For this review, use the dimensioned drawing (mm, ordinates from the lowest corner) and the shaded views. Round coordinates to 2 decimals unless told otherwise and drop trailing zeros. Write each loop counter-clockwise with the first axis right and the second up, starting at its lowest first coordinate (ties: lowest second). Pieces come first, ordered by that corner, then holes. Notation, with made-up numbers: M 27.5,34 L 79.5,34 A19 ccw 79.5,41 Z; hole C 21.5,78 d5. An arc over 180 degrees is marked long. One line per question, with ' | ' between items. Start each with the question number.
Item 1: For L1, parallel to Y at x = 2.25, z = 0.75 (1 decimal); L2, parallel to Z at x = 1, y = 1.5; L3, parallel to Z at x = 0.5, y = 2.25 (1 decimal), list the stretches that pass through material, from the lowest coordinate up.
Item 2: Insertion check: pin 1 Ø2.5 at (x, y) = (3.175, 3.175) entering from -Z; pin 2 Ø1 at (y, z) = (1, 2) entering from -X. Each pin has a flat end and moves straight along its axis. Give the tip position at first contact, or say it passes through.
Item 3: Add section B-B, the plane z = 2.55. State the section outline as (x, y) points (1 decimal).
Item 4: Add section A-A, the plane z = 1.75. State the section outline as (x, y) points (1 decimal).
Item 5: Draft analysis for pull direction Y (two halves, no side actions). For the marked faces 1, 2 and 3, state which applies: released by +Y, released by -Y, zero draft, split by the parting line, or undercut.
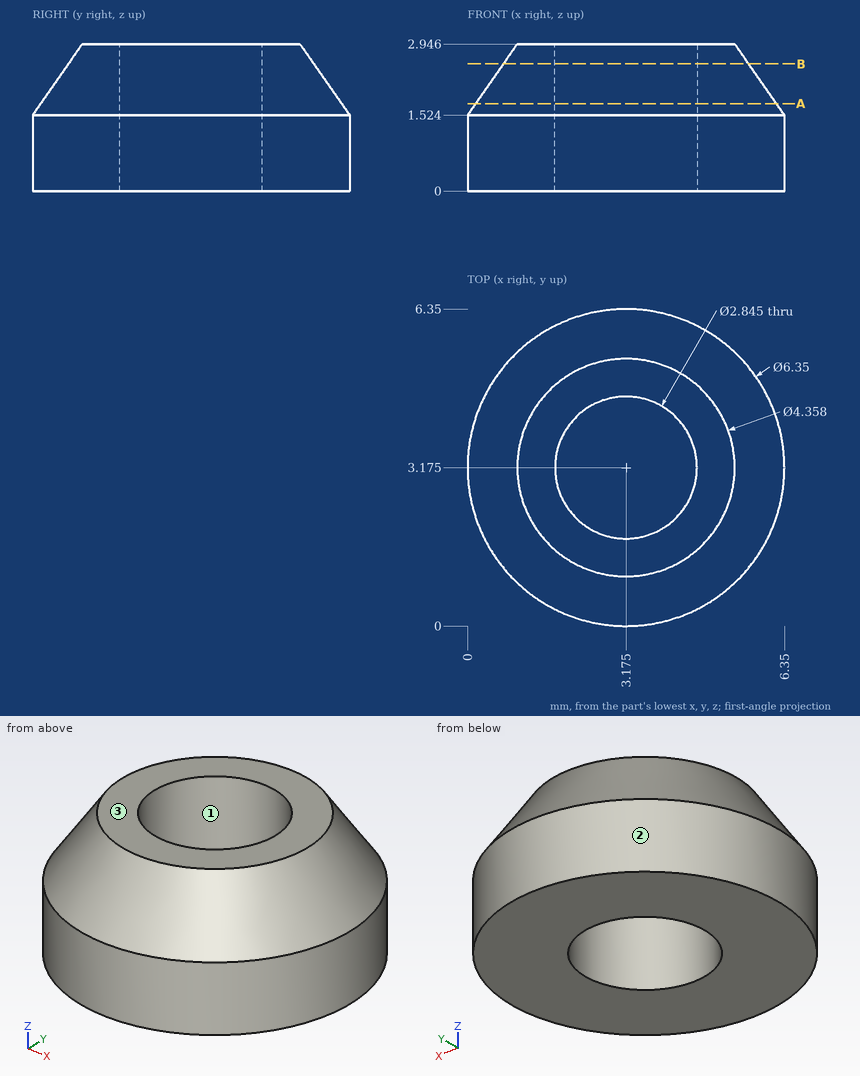
Computed values:
1) L1: y = 0.1 to 2.1, 4.3 to 6.2 | L2: z = 0 to 2.14 | L3: z = 0 to 2
2) pin 1: passes through | pin 2: stops at x = 0.68
3) outline: C 3.2,3.2 d4.9; hole C 3.2,3.2 d2.8
4) outline: C 3.2,3.2 d6; hole C 3.2,3.2 d2.8
5) face 1: undercut | face 2: split by the parting line | face 3: zero draft
